Source: three-view drawing plus pictorial views. Frame: mm from the lowest corner of the part. A direction names the side the tool comes from. Coordinates: 2 decimals unless noted, no trailing zeros. Loops run counter-clockwise (first coordinate to the right, second up) from the corner with the lowest first, then second, coordinate; pieces in that order, holes last. Notation, with made-up numbers: M 32.25,28.25 L 69.25,28.25 A15 ccw 69.25,47.25 Z; hole C 88.25,-4.5 d7. An arc over 180 degrees is marked long. Write each question's results on one line, items separated by ' | '. Start each with the question number.
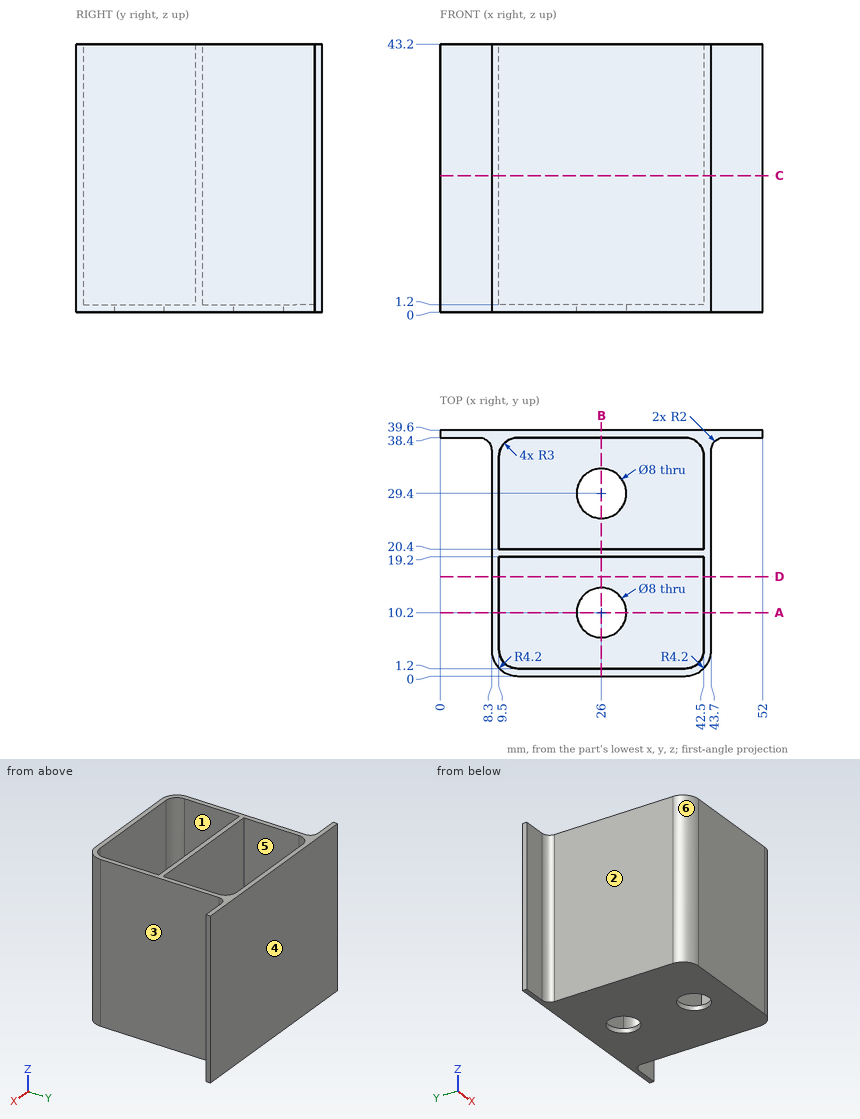
Item 1: Ray query, L1, parallel to Y at x = 27, z = 17; L2, parallel to Y at x = 26, z = 0.95; L3, parallel to X at y = 8.5, z = 7. Return the intervals inside material, ascending. Write a range as [from, to].
Item 2: Section C-C, the plane z = 22. Return loops of the section in (x, y).
Item 3: Contact query for flat-ended pins moving along their axis: P1, Ø3, axis at x = 49.5, z = 30.5, coming from the -Y side; P2, Ø10.5, axis at x = 26, y = 10.2, coming from the +Z side; P3, Ø4.5, axis at y = 13.5, z = 28, coming from the +X side; P4, Ø1, axis at x = 45.5, y = 7, coming from the +Z side. Output: stop coordinate, or through.
Item 4: Section D-D, the plane y = 16. Return loops of the section in (x, z).
Item 5: Section A-A, the plane y = 10.2. Return loops of the section in (x, z), plus the area to 3 significant figures.
Item 6: Set-up query: the marked faces 1, 2 and 3. Return all of +Z, -Z, +X, -X, +Y, -Y with unobstructed straight access to the full face (end or side cutting, diameter ignored); none if empty.
Item 7: Pull-direction query (Y, two-part tool) for the marked faces 4, 5 and 6; classes: released by +Y, released by -Y, zero draft, split by the parting line, or undercut.
Item 8: Section B-B, the plane x = 26. Return loops of the section in (y, z), plus the area to 3 significant figures.
Solutions:
1) L1: y = [0, 1.2], [19.2, 20.4], [38.4, 39.6] | L2: y = [0, 6.2], [14.2, 25.4], [33.4, 39.6] | L3: x = [8.3, 9.5], [42.5, 43.7]
2) outline: M 0,38.4 L 6.3,38.4 A2 cw 8.3,36.4 L 8.3,4.2 A4.2 ccw 12.5,0 L 39.5,0 A4.2 ccw 43.7,4.2 L 43.7,36.4 A2 cw 45.7,38.4 L 52,38.4 L 52,39.6 L 0,39.6 Z; hole M 9.5,4.2 A3 ccw 12.5,1.2 L 39.5,1.2 A3 ccw 42.5,4.2 L 42.5,19.2 L 9.5,19.2 Z; hole M 9.5,20.4 L 42.5,20.4 L 42.5,35.4 A3 ccw 39.5,38.4 L 12.5,38.4 A3 ccw 9.5,35.4 Z
3) P1: stops at y = 38.4 | P2: stops at z = 1.2 | P3: stops at x = 43.7 | P4: passes through
4) outline: M 8.3,0 L 43.7,0 L 43.7,43.2 L 42.5,43.2 L 42.5,1.2 L 9.5,1.2 L 9.5,43.2 L 8.3,43.2 Z
5) outline: M 8.3,0 L 22,0 L 22,1.2 L 9.5,1.2 L 9.5,43.2 L 8.3,43.2 Z; M 30,0 L 43.7,0 L 43.7,43.2 L 42.5,43.2 L 42.5,1.2 L 30,1.2 Z | area: 134 mm²
6) face 1: +Z | face 2: +Z, -Z, -X, -Y | face 3: +Z, -Z, +X, -Y
7) face 4: released by +Y | face 5: undercut | face 6: released by -Y
8) outline: M 0,0 L 6.2,0 L 6.2,1.2 L 1.2,1.2 L 1.2,43.2 L 0,43.2 Z; M 14.2,0 L 25.4,0 L 25.4,1.2 L 20.4,1.2 L 20.4,43.2 L 19.2,43.2 L 19.2,1.2 L 14.2,1.2 Z; M 33.4,0 L 39.6,0 L 39.6,43.2 L 38.4,43.2 L 38.4,1.2 L 33.4,1.2 Z | area: 180 mm²
